from build123d import *

# Parameters (mm, degrees)
SKETCH1_W           = 31.3
SKETCH1_H           = 20
BOSS_EXTRUDE1_DEPTH = 7
SKETCH2_W           = 31.3
SKETCH2_H           = 20
BOSS_EXTRUDE2_DEPTH = 1
BOSS_EXTRUDE4_START = -0.25
SKETCH3_W           = 29.3
SKETCH3_H           = 18
BOSS_EXTRUDE4_DEPTH = 5.75


with BuildPart() as part:
    # Sketch1 → Boss-Extrude1 (new body)
    with BuildSketch(Plane(origin=(0, 0, 0), x_dir=(1, 0, 0), z_dir=(0, 1, 0))):
        Rectangle(SKETCH1_W, SKETCH1_H)
        Polygon((-14.65, -9), (-14.65, 9), (-7, 9), (-7, 7), (-6, 7), (-6, 9), (6, 9), (6, 7), (7, 7), (7, 9), (14.65, 9), (14.65, -9), (7, -9), (7, -7), (6, -7), (6, -9), (-6, -9), (-6, -7), (-7, -7), (-7, -9), align=None, mode=Mode.SUBTRACT)
    extrude(amount=BOSS_EXTRUDE1_DEPTH)

    # Sketch2 → Boss-Extrude2 (add)
    with BuildSketch(Plane(origin=(0, 7, 0), x_dir=(1, 0, 0), z_dir=(0, 1, 0))):
        Rectangle(SKETCH2_W, SKETCH2_H)
    extrude(amount=-BOSS_EXTRUDE2_DEPTH)

    # Sketch3 → Boss-Extrude4 (add)
    with BuildSketch(Plane.XZ.offset(BOSS_EXTRUDE4_START)):
        Rectangle(SKETCH3_W, SKETCH3_H)
    extrude(amount=-BOSS_EXTRUDE4_DEPTH)


solid = part.part
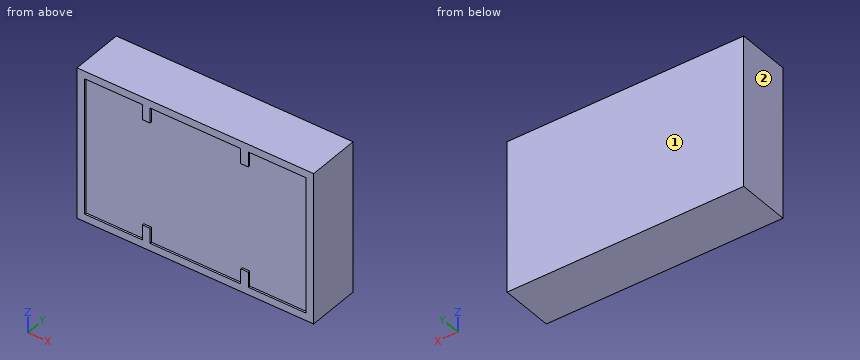
Verification items for the finished model (mm, model axes). Face numbers are marked on the shaded views. Round coordinates to 2 decimals unless told otherwise and drop trailing zeros. Loops run counter-clockwise (first coordinate to the right, second up) from the corner with the lowest first, then second, coordinate; pieces in that order, holes last. Notation, with made-up numbers: (44, 55.5) - (69, 55.5) arc R28 cw to (69, 91.5) - close; hole circle Ø5 at (-35, 22.25). An arc over 180 degrees is marked (long way). Answer in a Markdown table with one row per item. Add a question column.
Q1. Material ranges on line 1 (Y direction, x = 6.5, z = -2.75), recorded low to high.
Q2. Release check for a two-part mould opening along Y. For the marked faces 1 and 2 record: pulls with the +Y half, pulls with the -Y half, needs draft (parallel to the pull), parting line crosses it, or undercut.
Q3. Section check B-B on x = 8. Enter the section's corners in (y, z).
Q4. Section check A-A on z = -2.75. Enter the section's corners in (x, y), plus the area to 3 significant figures.
Q5. Gauge pin test, flat end, axial feed: pin 1 (1.5 mm diameter, centred on x = 2.5, z = -5, fed in from -Y). Record the tip position at first contact, or that the pin passes through.
Found:
| question | item | result |
|---|---|---|
| 1 | line 1 | y = 0.25 to 7 |
| 2 | face 1 | pulls with the +Y half |
| 2 | face 2 | needs draft |
| 3 | outline | (0, -10) - (7, -10) - (7, 10) - (0, 10) - (0, 9) - (0.25, 9) - (0.25, -9) - (0, -9) - close |
| 4 | outline | (-15.65, 0) - (-14.65, 0) - (-14.65, 0.25) - (14.65, 0.25) - (14.65, 0) - (15.65, 0) - (15.65, 7) - (-15.65, 7) - close |
| 4 | area | 212 mm² |
| 5 | pin 1 | stops at y = 0.25 |
